from build123d import *

# Parameters (mm, degrees)
F0_W     = 56
F0_H     = 56
F1_DEPTH = 12
F2_R     = 22.5
F3_DEPTH = 12
F5_D     = 4.7
F6_R     = 4.5


with BuildPart() as f1:
    # F0 (on Top) → F1 (new body)
    with BuildSketch(Plane.XY):
        with Locations((28, 28)):
            Rectangle(F0_W, F0_H)
    extrude(amount=F1_DEPTH)

    # F2 (on face) → F3 (cut, through all)
    with BuildSketch(Plane.XY.offset(12)):
        with Locations((28, 28)):
            Circle(F2_R)
    extrude(amount=-F3_DEPTH, mode=Mode.SUBTRACT)

    # F5 (through all)
    with Locations(Plane.XY.offset(12)):
        with Locations((4.43, 51.57), (51.57, 51.57), (51.57, 4.43), (4.43, 4.43)):
            Hole(F5_D / 2)

    # F6
    f6_edges = [f1.edges().sort_by_distance(p)[0] for p in [
        (56, 56, 6),
        (56, 0, 6),
        (0, 0, 6),
        (0, 56, 6),
    ]]
    fillet(f6_edges, radius=F6_R)


solid = f1.part
Build history of the part. All positions in model axes, mm. Round coordinates to 2 decimals unless told otherwise and drop trailing zeros. Write each loop counter-clockwise with the first axis right and the second up, starting at its lowest first coordinate (ties: lowest second). Pieces come first, ordered by that corner, then holes. Notation, with made-up numbers: (85, 3.25) - (134, 3.25) arc R31 cw to (134, 33.25) - close; hole circle Ø5 at (69, 6.25). An arc over 180 degrees is marked (long way). Use CSV: the item, a comma, the result in double quotes.
(1) Wall check: line 1 (X direction, y = 4.5, z = 1.25); line 2 (Y direction, x = 28, z = 9.25). Give the ranges that are in metal, low to high.
Response:
line 1,"0 to 2.08, 6.78 to 49.22, 53.92 to 56"
line 2,"0 to 5.5, 50.5 to 56"
(2) Band-saw the part on B-B (x = 28). Write the cut outline in (y, z), plus the area to 3 significant figures.
Response:
outline,"(0, 0) - (5.5, 0) - (5.5, 12) - (0, 12) - close; (50.5, 0) - (56, 0) - (56, 12) - (50.5, 12) - close"
area,"132 mm²"
(3) Pin check, flat tip, straight feed: P1, Ø4, axis at x = 17.5, y = 8.5, coming from the +Z side. Stop position of the tip, or through.
Response:
P1,"z = 12"
(4) Mould opens along Y. For faces 1 (the cylindrical face through (3.346, 2.345, 5.916)), 2 (the cylindrical face through (54.647, 1.283, 6.084)), 3 (the flat face through (15, 47, 12)) say: pulls with the +Y half, pulls with the -Y half, needs draft (parallel to the pull), parting line crosses it, or undercut.
Response:
face 1,"undercut"
face 2,"pulls with the -Y half"
face 3,"needs draft"
(5) Band-saw the part on C-C (y = 14.5). Write the cut outline in (x, z).
Response:
outline,"(0, 0) - (10, 0) - (10, 12) - (0, 12) - close; (46, 0) - (56, 0) - (56, 12) - (46, 12) - close"
(6) Band-saw the part on A-A (z = 11.25). Write the cut outline in (x, y).
Response:
outline,"(0, 4.5) arc R4.5 ccw to (4.5, 0) - (51.5, 0) arc R4.5 ccw to (56, 4.5) - (56, 51.5) arc R4.5 ccw to (51.5, 56) - (4.5, 56) arc R4.5 ccw to (0, 51.5) - close; hole circle Ø4.7 at (4.43, 4.43); hole circle Ø4.7 at (4.43, 51.57); hole circle Ø45 at (28, 28); hole circle Ø4.7 at (51.57, 4.43); hole circle Ø4.7 at (51.57, 51.57)"
